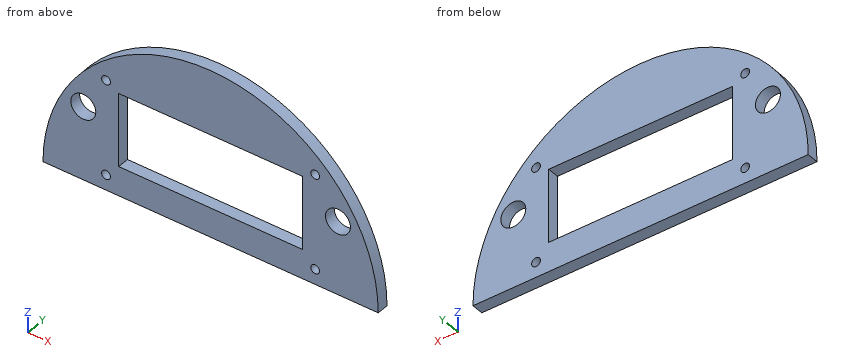
```python
from build123d import *

# Parameters (mm, degrees)
ESQUISSE1_R             = 4.25
ESQUISSE1_W             = 62.5
ESQUISSE1_H             = 25
BOSS_EXTRU_1_DEPTH      = 4
ESQUISSE2_R             = 1.5
ENL_V_MAT_EXTRU_1_DEPTH = 81.709355096


with BuildPart() as part:
    # Esquisse1 → Boss.-Extru.1 (new body)
    with BuildSketch(Plane(origin=(0, 0, 0), x_dir=(1, 0, 0), z_dir=(0, 1, 0))):
        with BuildLine():
            Line((-57, 0), (57, 0))
            ThreePointArc((57, 0), (0, -57), (-57, 0))
        make_face()
        with Locations(Location((-43.301270189, -25, 0), (0, 0, 270))):
            Circle(ESQUISSE1_R, mode=Mode.SUBTRACT)
        with Locations(Location((43.301270189, -25, 0), (0, 0, 270))):
            Circle(ESQUISSE1_R, mode=Mode.SUBTRACT)
        with Locations((0, -22.5)):
            Rectangle(ESQUISSE1_W, ESQUISSE1_H, mode=Mode.SUBTRACT)
    extrude(amount=BOSS_EXTRU_1_DEPTH)

    # Esquisse2 → Enlèv. mat.-Extru.1 (cut, through all)
    with BuildSketch(Plane(origin=(0, 4, 0), x_dir=(1, 0, 0), z_dir=(0, 1, 0))):
        with Locations(Location((-35.557071612, -37.554578926, 0), (0, 0, 270))):
            Circle(ESQUISSE2_R)
        with Locations(Location((-35.557071612, -5.198506408, 0), (0, 0, 270))):
            Circle(ESQUISSE2_R)
        with Locations(Location((35.557071612, -5.198506408, 0), (0, 0, 270))):
            Circle(ESQUISSE2_R)
        with Locations(Location((35.557071612, -37.554578926, 0), (0, 0, 270))):
            Circle(ESQUISSE2_R)
    extrude(amount=-ENL_V_MAT_EXTRU_1_DEPTH, mode=Mode.SUBTRACT)


solid = part.part
```
For this review, take the finished solid that the model builds, in its own axes (mm). Round coordinates to 2 decimals unless told otherwise and drop trailing zeros. Loops run counter-clockwise (first coordinate to the right, second up) from the corner with the lowest first, then second, coordinate; pieces in that order, holes last.
(1) We need section A-A (x = 0). Give the boundary of the cut face in (y, z).
Returned:
outline: (0, 0) - (4, 0) - (4, 10) - (0, 10) - close; (0, 35) - (4, 35) - (4, 57) - (0, 57) - close
(2) We need section C-C (y = 1.35). Give the boundary of the cut face in (x, z), plus the area to 3 significant figures.
Returned:
outline: (-57, 0) - (57, 0) arc R57 ccw to start; hole circle Ø8.5 at (-43.3, 25); hole circle Ø3 at (-35.56, 5.2); hole circle Ø3 at (-35.56, 37.55); hole (-31.25, 10) - (31.25, 10) - (31.25, 35) - (-31.25, 35) - close; hole circle Ø3 at (35.56, 5.2); hole circle Ø3 at (35.56, 37.55); hole circle Ø8.5 at (43.3, 25)
area: 3,400 mm2
(3) Wall thickness on line 1 along Z through (x, y) = (1, 1.1); line 2 along Z through (x, y) = (35, 1.3); line 3 along X through (y, z) = (2.45, 6): over which ranges is each line inside the solid? List them lowest first.
Returned:
line 1: z = 0 to 10, 35 to 56.99
line 2: z = 0 to 3.81, 6.59 to 36.16, 38.95 to 44.99
line 3: x = -56.68 to -36.82, -34.29 to 34.29, 36.82 to 56.68
(4) Clearance check with flat-ended pins moving along their axes: P1, Ø1.2, axis at y = 1.5, z = 22.5, coming from the +X side (3 decimals); P2, Ø1.5, axis at y = 2, z = 8, coming from the -X side; P3, Ø1.2, axis at y = 1, z = 19.5, coming from the -X side. State where each tip first meets the part, or that it passes through.
Returned:
P1: stops at x = 52.625
P2: stops at x = -56.54
P3: stops at x = -53.78
(5) We need section D-D (z = 18). Give the boundary of the cut face in (x, y).
Returned:
outline: (-54.08, 0) - (-31.25, 0) - (-31.25, 4) - (-54.08, 4) - close; (31.25, 0) - (54.08, 0) - (54.08, 4) - (31.25, 4) - close
(6) We need section B-B (z = 25). Give the boundary of the cut face in (x, y) (3 decimals).
Returned:
outline: (-51.225, 0) - (-47.551, 0) - (-47.551, 4) - (-51.225, 4) - close; (-39.051, 0) - (-31.25, 0) - (-31.25, 4) - (-39.051, 4) - close; (31.25, 0) - (39.051, 0) - (39.051, 4) - (31.25, 4) - close; (47.551, 0) - (51.225, 0) - (51.225, 4) - (47.551, 4) - close
